Drawing for the job (mm, zero at the part's lowest x, y, z). Coordinates: 2 decimals unless noted, no trailing zeros. Loops run counter-clockwise (first coordinate to the right, second up) from the corner with the lowest first, then second, coordinate; pieces in that order, holes last. Notation, with made-up numbers: (64, 45.25) -> (116, 45.25) arc R16 ccw to (116, 54.25) -> close; hole circle Ø5 at (-10, -27.75). An arc over 180 degrees is marked (long way). Write item = value, one per line. Start each with the question number.
(1) Flat gauge pins, fed straight in: P1, Ø1.5, axis at x = 87.5, y = 1, coming from the -Z side (1 decimal); P2, Ø1.5, axis at y = 1.5, z = 52.5, coming from the -X side; P3, Ø1.5, axis at y = 1, z = 11, coming from the -X side. Where does each tip first touch, or does it go through?
(2) Band-saw the part on A-A (z = 12.5). Write the cut outline in (x, y).
(3) Band-saw the part on C-C (x = 88.5). Write the cut outline in (y, z), and give its area (3 significant figures).
(4) Band-saw the part on B-B (y = 2.05). Write the cut outline in (x, z) (3 decimals).
(5) Drill centre lines: line 1 (X direction, y = 2.75, z = 51); line 2 (X direction, y = 2.9, z = 19.5); line 3 (X direction, y = 1.85, z = 50). Where is each one in solid material? Low to high. Write a range as from..to.
(6) Band-saw the part on D-D (z = 24). Write the cut outline in (x, y).
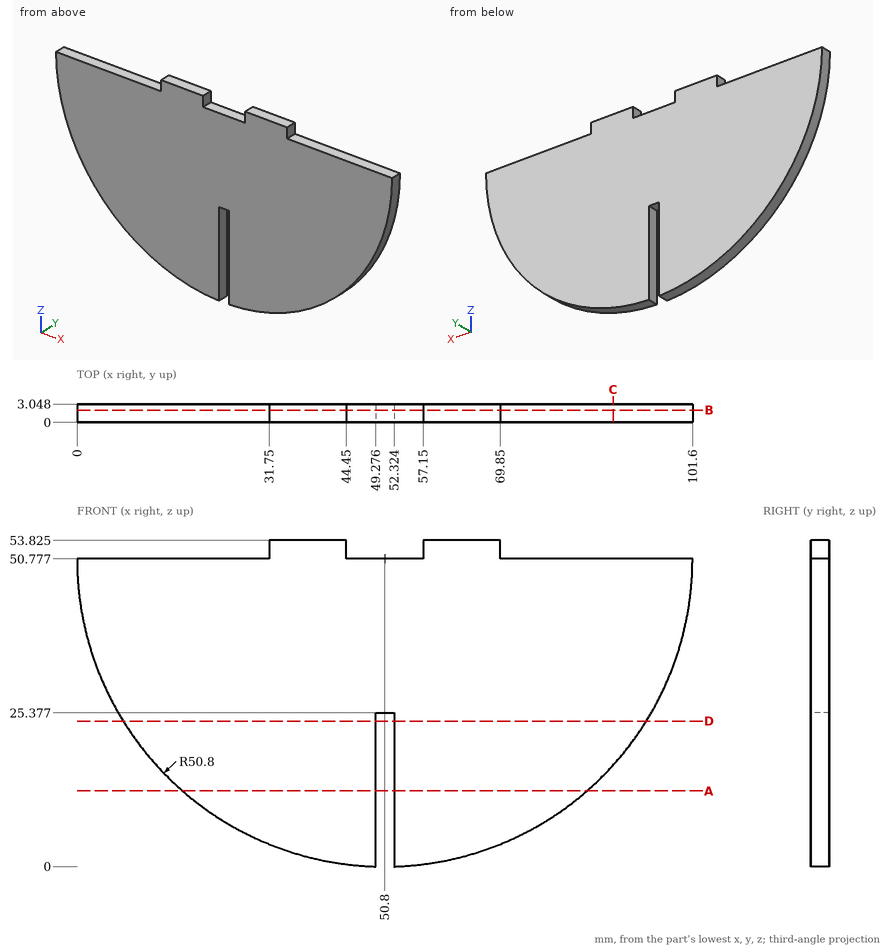
Findings below:
q1.P1 = 14.9
q1.P2 = 31.75
q1.P3 = 18.28
q2.outline = (17.4, 0) -> (49.28, 0) -> (49.28, 3.05) -> (17.4, 3.05) -> close; (52.32, 0) -> (84.2, 0) -> (84.2, 3.05) -> (52.32, 3.05) -> close
q3.outline = (0, 16.73) -> (3.05, 16.73) -> (3.05, 50.78) -> (0, 50.78) -> close
q3.area = 104 mm²
q4.outline = (0, 50.777) arc R50.8 ccw to (49.276, 0) -> (49.276, 25.377) -> (52.324, 25.377) -> (52.324, 0) arc R50.8 ccw to (101.6, 50.777) -> (69.85, 50.777) -> (69.85, 53.825) -> (57.15, 53.825) -> (57.15, 50.777) -> (44.45, 50.777) -> (44.45, 53.825) -> (31.75, 53.825) -> (31.75, 50.777) -> close
q5.line_1 = 31.75..44.45, 57.15..69.85
q5.line_2 = 10.77..49.28, 52.32..90.83
q5.line_3 = 0.01..101.59
q6.outline = (7.63, 0) -> (49.28, 0) -> (49.28, 3.05) -> (7.63, 3.05) -> close; (52.32, 0) -> (93.97, 0) -> (93.97, 3.05) -> (52.32, 3.05) -> close
